```python
from build123d import *

# Parameters (mm, degrees)
F0_R     = 9
F1_DEPTH = 24
F2_R     = 4.1
F3_DEPTH = 12
F4_R     = 2.6
F5_DEPTH = 25
F6_R     = 1.5
F7_DEPTH = 25


with BuildPart() as f1:
    # F0 (on Top) → F1 (new body)
    with BuildSketch(Plane.XY):
        Circle(F0_R)
    extrude(amount=F1_DEPTH)

    # F2 (on face) → F3 (cut)
    with BuildSketch(Plane.XY.offset(24)):
        Circle(F2_R)
    extrude(amount=-F3_DEPTH, mode=Mode.SUBTRACT)

    # F4 (on face) → F5 (cut)
    with BuildSketch(Plane(origin=(0, 0, 0), x_dir=(1, 0, 0), z_dir=(0, 0, -1))):
        Circle(F4_R)
    extrude(amount=-F5_DEPTH, mode=Mode.SUBTRACT)

    # F6 (on Right) → F7 (cut)
    with BuildSketch(Plane.YZ):
        with Locations((0, 17)):
            Circle(F6_R)
        with Locations((0, 7)):
            Circle(F6_R)
    extrude(amount=-F7_DEPTH, mode=Mode.SUBTRACT)


solid = f1.part
```
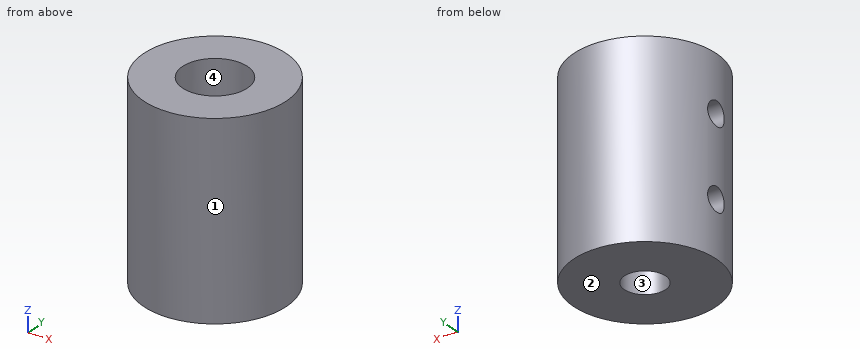
Here's how the part is built. I have some questions about the finished solid (model axes, mm). Face numbers are marked on the shaded views. Round coordinates to 2 decimals unless told otherwise and drop trailing zeros. Write each loop counter-clockwise with the first axis right and the second up, starting at its lowest first coordinate (ties: lowest second). Pieces come first, ordered by that corner, then holes. Notation, with made-up numbers: M 43,-30.5 L 81,-30.5 A25 cw 81,-6.5 Z; hole C 88,-2.5 d7. An arc over 180 degrees is marked long. Answer as CSV lines item,"result". Start each with the question number.
1. Suppose I cut it at A-A on y = 0. Write out the boundary of the cut face in (x, z).
2. Suppose I cut it at B-B on x = 0. Write out the boundary of the cut face in (y, z).
3. I need wall thicknesses on probe 1 along Y at (x, z) = (0, 15.75); probe 2 along Y at (x, z) = (-1, 8.25); probe 3 along X at (y, z) = (0, 16.75). Which ranges of each line are inside material? Lowest first, please.
4. I'm going to push flat-ended pins straight in: pin 1 Ø2 at (y, z) = (2.5, 20) entering from +X; pin 2 Ø4 at (x, z) = (-7, 14.5) entering from +Y; pin 3 Ø9 at (x, y) = (-2, 0) entering from +Z; pin 4 Ø5 at (x, z) = (3.5, 3) entering from -Y. Where does each tip first touch, or does it pass through?
5. Suppose I cut it at D-D on z = 5. Write out the boundary of the cut face in (x, y).
6. Thinking about a two-plate mould opening in X: for the marked faces 1, 2, 3 and 4, which applies, released by +X, released by -X, zero draft, split by the parting line, or undercut?
7. Suppose I cut it at C-C on y = 2. Write out the boundary of the cut face in (x, z).
Check result:
1,outline,"M -9,0 L -2.6,0 L -2.6,5.5 L -9,5.5 Z; M -9,8.5 L -2.6,8.5 L -2.6,12 L -4.1,12 L -4.1,15.5 L -9,15.5 Z; M -9,18.5 L -4.1,18.5 L -4.1,24 L -9,24 Z; M 2.6,0 L 9,0 L 9,24 L 4.1,24 L 4.1,12 L 2.6,12 Z"
2,outline,"M -9,0 L -2.6,0 L -2.6,12 L -4.1,12 L -4.1,24 L -9,24 Z; M 2.6,0 L 9,0 L 9,24 L 4.1,24 L 4.1,12 L 2.6,12 Z"
3,probe 1,"y = -9 to -4.1, 4.1 to 9"
3,probe 2,"y = -8.94 to -2.4, 2.4 to 8.94"
3,probe 3,"x = 4.1 to 9"
4,pin 1,"stops at x = 8.87"
4,pin 2,"stops at y = 7.48"
4,pin 3,"stops at z = 24"
4,pin 4,"stops at y = -8.94"
5,outline,"C 0,0 d18; hole C 0,0 d5.2"
6,face 1,"split by the parting line"
6,face 2,"zero draft"
6,face 3,"undercut"
6,face 4,"undercut"
7,outline,"M -8.77,0 L -1.66,0 L -1.66,12 L -3.58,12 L -3.58,24 L -8.77,24 Z; M 1.66,0 L 8.77,0 L 8.77,24 L 3.58,24 L 3.58,12 L 1.66,12 Z"
